Design review of the part built by this model. Coordinates are the model's own, in mm. Face numbers are marked on the shaded views. Coordinates: 2 decimals unless noted, no trailing zeros. Loops run counter-clockwise (first coordinate to the right, second up) from the corner with the lowest first, then second, coordinate; pieces in that order, holes last. Notation, with made-up numbers: (-14.75, -12.5) -> (41.25, -12.5) arc R14 ccw to (41.25, -5.5) -> close; hole circle Ø5 at (1, 5.25). An arc over 180 degrees is marked (long way). Use CSV: the item, a comma, the result in double quotes.
Autodesk Inventor part; units mm, degrees
ref_plane "YZ Plane" through (0, 0, 0) normal (1, 0, 0) x (0, 1, 0)
ref_plane "XZ Plane" through (0, 0, 0) normal (0, 1, 0) x (-1, 0, 0)
ref_plane "XY Plane" through (0, 0, 0) normal (0, 0, 1) x (1, 0, 0)
sketch "Sketch1" plane through (0, 0, 0) normal (0, 1, 0) x (-1, 0, 0)
  line L0 (-5.5, 3.1754) -> (0, 6.3509)
  line L1 (0, 6.3509) -> (5.5, 3.1754)
  line L2 (5.5, 3.1754) -> (5.5, -3.1754)
  line L3 (5.5, -3.1754) -> (0, -6.3509)
  line L4 (0, -6.3509) -> (-5.5, -3.1754)
  line L5 (-5.5, -3.1754) -> (-5.5, 3.1754)
  line L6 (0, 7.2373) -> (0, -7.2373)
  point P0 (0, 0)
  point P1 (0, 0)
  point P2 (0, 0)
  point P3 (0, 0)
  dimension "d0" = 11
extrude "Extrusion1" add sketch "Sketch1" along normal blind 4
hole "Hole1" at (0, 0, 0) direction (0, 1, 0) diameter 8 end through all
thread "Thread1"
properties part number "HUDSON-1-79"
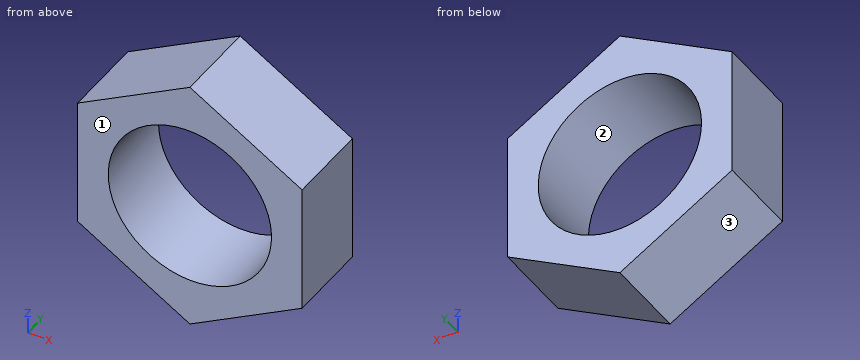
Item 1: Clearance check with a flat-ended pin moving along its axis: pin 1 (5 mm diameter, centred on x = 0, z = 0, fed in from +Y). State where the tip first meets the part, or that it passes through.
Checked values:
pin 1,"through"
Item 2: To check wall thickness, follow line 1 along X through (y, z) = (2.15, 0); line 2 along Z through (x, y) = (1.75, 0.9); line 3 along X through (y, z) = (2.65, 0.75). State the ranges of each line that lie inside material, in increasing order.
Checked values:
line 1,"-5.5 to -4, 4 to 5.5"
line 2,"-5.34 to -3.6, 3.6 to 5.34"
line 3,"-5.5 to -3.93, 3.93 to 5.5"
Item 3: Draft analysis for pull direction Z (two halves, no side actions). For the marked faces 1, 2 and 3, state which applies: pulls with the +Z half, pulls with the -Z half, needs draft (parallel to the pull), parting line crosses it, or undercut.
Checked values:
face 1,"needs draft"
face 2,"undercut"
face 3,"pulls with the -Z half"
Item 4: Add section B-B (x = -2.5). Give the boundary of the cut face in (y, z), then the cut area to 3 significant figures.
Checked values:
outline,"(0, -4.91) -> (4, -4.91) -> (4, -3.12) -> (0, -3.12) -> close; (0, 3.12) -> (4, 3.12) -> (4, 4.91) -> (0, 4.91) -> close"
area,"14.3 mm^2"
Item 5: Add section A-A (z = 0). Give the boundary of the cut face in (x, y), then the cut area to 3 significant figures.
Checked values:
outline,"(-5.5, 0) -> (-4, 0) -> (-4, 4) -> (-5.5, 4) -> close; (4, 0) -> (5.5, 0) -> (5.5, 4) -> (4, 4) -> close"
area,"12.0 mm^2"
Item 6: Add section D-D (z = -4.5). Give the boundary of the cut face in (x, y), then the cut area to 3 significant figures.
Checked values:
outline,"(-3.21, 0) -> (3.21, 0) -> (3.21, 4) -> (-3.21, 4) -> close"
area,"25.6 mm^2"
Item 7: Add section C-C (y = 3.15). Give the boundary of the cut face in (x, z), then the cut area to 3 significant figures.
Checked values:
outline,"(-5.5, -3.18) -> (0, -6.35) -> (5.5, -3.18) -> (5.5, 3.18) -> (0, 6.35) -> (-5.5, 3.18) -> close; hole circle Ø8 at (0, 0)"
area,"54.5 mm^2"
